The model under review builds one solid part; all positions refer to its coordinate system, in mm. A direction names the side the tool comes from. Round coordinates to 2 decimals unless told otherwise and drop trailing zeros. Write each loop counter-clockwise with the first axis right and the second up, starting at its lowest first coordinate (ties: lowest second). Pieces come first, ordered by that corner, then holes. Notation, with made-up numbers: (-18.5, -27.5) - (13.5, -27.5) arc R25 ccw to (13.5, 2.5) - close; hole circle Ø6 at (74, -14). An arc over 180 degrees is marked (long way). Use one line per item in the form item = value.
from build123d import *

# Parameters (mm, degrees)
SKETCH1_R           = 42.164
SKETCH1_R_2         = 29.464
BOSS_EXTRUDE1_DEPTH = 164.973
SKETCH2_R           = 9.525
BOSS_EXTRUDE2_DEPTH = 19.84375


with BuildPart() as part:
    # Sketch1 → Boss-Extrude1 (new, symmetric)
    with BuildSketch(Plane(origin=(0, 0, 0), x_dir=(1, 0, 0), z_dir=(0, 1, 0))):
        with Locations(Location((0, 0, 0), (0, 0, 90))):
            Circle(SKETCH1_R)
        with Locations(Location((0, 0, 0), (0, 0, 90))):
            Circle(SKETCH1_R_2, mode=Mode.SUBTRACT)
    extrude(amount=BOSS_EXTRUDE1_DEPTH, both=True)

    # Sketch2 → Boss-Extrude2 (add, symmetric)
    with BuildSketch(Plane.XY):
        with BuildLine():
            Line((-63.646931448, -157.056172579), (-42.164, -164.973))
            Line((-42.164, -164.973), (-29.464, -164.973))
            Line((-29.464, -164.973), (-29.464, 9.158002397))
            Line((-29.464, 9.158002397), (-78.697172579, -124.440068552))
            ThreePointArc((-78.697172579, -124.440068552), (-77.927068333, -143.865127562), (-63.646931448, -157.056172579))
        make_face()
        with Locations(Location((-54.864, -133.223, 0), (0, 0, 180))):
            Circle(SKETCH2_R, mode=Mode.SUBTRACT)
    extrude(amount=BOSS_EXTRUDE2_DEPTH, both=True)


solid = part.part
(1) Add section A-A on x = 0. Write out the cut boundary in (y, z), then the cut area to 3 significant figures.
Geometry results:
outline = (-164.97, -42.16) - (164.97, -42.16) - (164.97, -29.46) - (-164.97, -29.46) - close; (-164.97, 29.46) - (164.97, 29.46) - (164.97, 42.16) - (-164.97, 42.16) - close
area = 8,380 mm2
(2) Machinability: for faces 5 (the flat face through (-54, -104, 19.844)), 6 (the flat face through (9, 164.973, 29)), 7 (the flat face through (-54, -104, -19.844)), which of the approach directions +Z, -Z, +X, -X, +Y, -Y give a long, thin tool a straight path to every point of the face, cutting with its end or side? Answer none if there is none.
Geometry results:
face_5 = +Z, -X, +Y, -Y
face_6 = +Z, -Z, +X, -X, +Y
face_7 = -Z, -X, +Y, -Y
(3) To check wall thickness, follow L1, parallel to X at y = -69, z = 0; L2, parallel to Z at x = -21, y = -68; L3, parallel to Z at x = 8, y = -75. State the ranges of each line that lie inside material, in increasing order.
Geometry results:
L1 = -58.27 to -29.46, 29.46 to 42.16
L2 = -36.56 to -20.67, 20.67 to 36.56
L3 = -41.4 to -28.36, 28.36 to 41.4
(4) Add section C-C on y = 5. Write out the cut boundary in (x, z), then the cut area to 3 significant figures.
Geometry results:
outline = circle Ø84.33 at (0, 0); hole circle Ø58.93 at (0, 0)
area = 2,860 mm2
(5) Insertion check: P1, Ø8, axis at y = 89, z = -22, coming from the +X side; P2, Ø5, axis at y = 95, z = -5, coming from the +X side; P3, Ø4, axis at y = 22.5, z = -14.5, coming from the +X side; P4, Ø15, axis at x = -54.864, y = -133.223, coming from the -Z side (1 decimal). Each pin has a flat end and moves straight along its axis. Give the tip position at first contact, or say it passes through.
Geometry results:
P1 = 38.13
P2 = 42.09
P3 = 40.27
P4 = through
(6) The part is to be moulded in two halves that separate along X. For faces 1 (the flat face through (-29, -164.973, -9)), 2 (the cylindrical face through (-53.624, -142.667, -0.278)), 3 (the cylindrical face through (41.16, 2.31, 9.14)), 4 (the flat face through (-53.056, -160.959, 0.278)), say which applies: +X half, -X half, draft (parallel to the pull), parting line (faces both ways), or undercut.
Geometry results:
face_1 = draft
face_2 = undercut
face_3 = parting line
face_4 = -X half
(7) Add section D-D on z = -11. Write out the cut boundary in (x, y) (3 decimals), then the cut area to 3 significant figures.
Geometry results:
outline = (-78.697, -124.44) arc R25.4 ccw to (-63.647, -157.056) - (-42.164, -164.973) - (-27.334, -164.973) - (-27.334, 164.973) - (-40.704, 164.973) - (-40.704, -21.342) - close; (27.334, -164.973) - (40.704, -164.973) - (40.704, 164.973) - (27.334, 164.973) - close; hole circle Ø19.05 at (-54.864, -133.223)
area = 11,800 mm2
(8) Add section B-B on z = 5. Write out the cut boundary in (x, y) (3 decimals).
Geometry results:
outline = (-78.697, -124.44) arc R25.4 ccw to (-63.647, -157.056) - (-42.164, -164.973) - (-29.037, -164.973) - (-29.037, 164.973) - (-41.866, 164.973) - (-41.866, -24.497) - close; (29.037, -164.973) - (41.866, -164.973) - (41.866, 164.973) - (29.037, 164.973) - close; hole circle Ø19.05 at (-54.864, -133.223)
